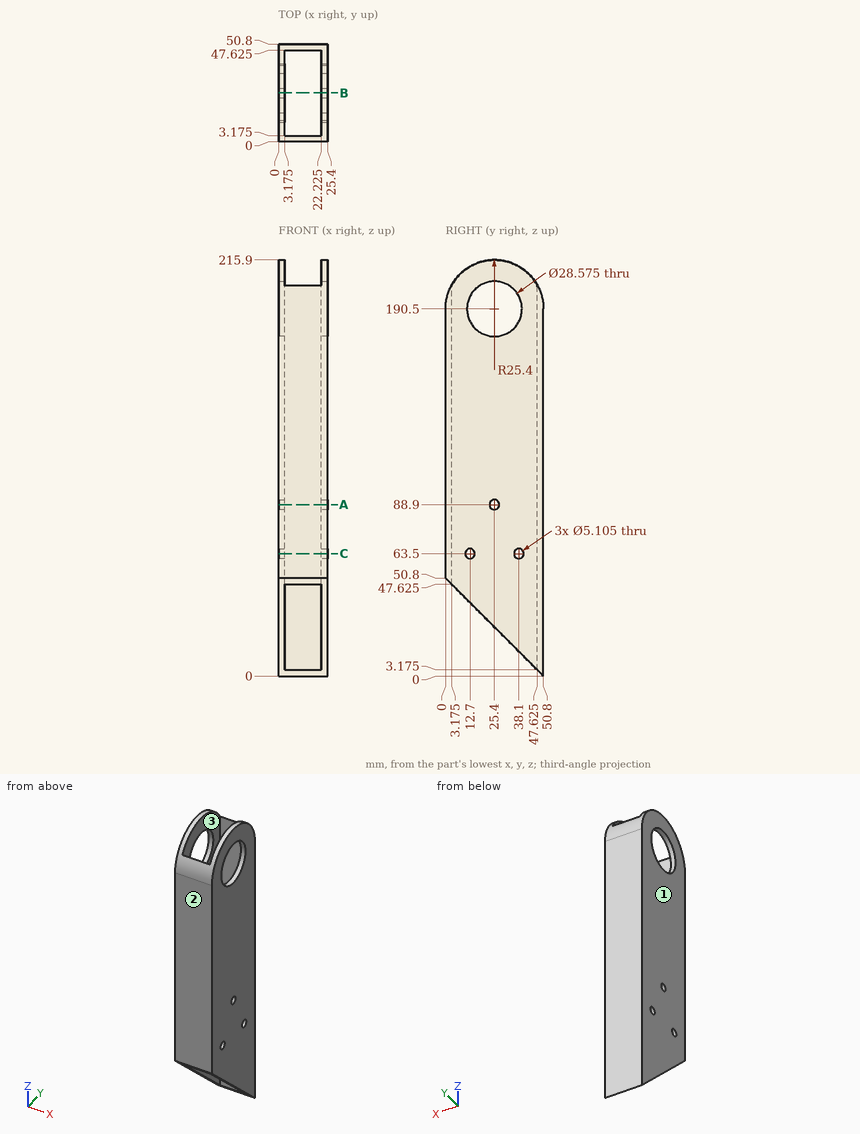
Input: dimensioned drawing with shaded views. Units: mm. Origin: part minimum x, y, z. Coordinates: 2 decimals unless noted, no trailing zeros. Loops run counter-clockwise (first coordinate to the right, second up) from the corner with the lowest first, then second, coordinate; pieces in that order, holes last. Notation, with made-up numbers: (-40, 64.5) -> (5, 64.5) arc R35 ccw to (5, 97.5) -> close; hole circle Ø5 at (66.25, 5.5). An arc over 180 degrees is marked (long way). Use a Markdown table: item, result. Add a question column.
(1) Section query A-A, the plane z = 88.9. Return loops of the section in (x, y) (1 decimal).
(2) Section query C-C, the plane z = 63.5. Return loops of the section in (x, y) (1 decimal).
(3) Section query B-B, the plane y = 25.4. Return loops of the section in (x, z) (1 decimal).
(4) Line query: line 1 along Y through (x, z) = (14.5, 163) (1 decimal); line 2 along X through (y, z) = (24, 168.5) (1 decimal); line 3 along Y through (x, z) = (0.65, 63.5). Output: solid intervals per line, ascending.
(5) Pin query (flat end, axial travel): pin 1 Ø8 at (y, z) = (12.7, 63.5) entering from +X; pin 2 Ø4 at (y, z) = (25.4, 88.9) entering from -X; pin 3 Ø2 at (x, y) = (21.5, 35) entering from -Z. Return the tip coordinate at first contact, or that it passes through.
(6) Mould query, pull axis Y, two halves, no side actions, for the marked faces 1, 2 and 3. Classes: pulls with the +Y half, pulls with the -Y half, needs draft (parallel to the pull), parting line crosses it, or undercut.
Answer:
| question | item | result |
|---|---|---|
| 1 | outline | (0, 0) -> (25.4, 0) -> (25.4, 22.8) -> (22.2, 22.8) -> (22.2, 3.2) -> (3.2, 3.2) -> (3.2, 22.8) -> (0, 22.8) -> close; (0, 28) -> (3.2, 28) -> (3.2, 47.6) -> (22.2, 47.6) -> (22.2, 28) -> (25.4, 28) -> (25.4, 50.8) -> (0, 50.8) -> close |
| 2 | outline | (0, 0) -> (25.4, 0) -> (25.4, 10.1) -> (22.2, 10.1) -> (22.2, 3.2) -> (3.2, 3.2) -> (3.2, 10.1) -> (0, 10.1) -> close; (0, 15.3) -> (3.2, 15.3) -> (3.2, 35.5) -> (0, 35.5) -> close; (0, 40.7) -> (3.2, 40.7) -> (3.2, 47.6) -> (22.2, 47.6) -> (22.2, 40.7) -> (25.4, 40.7) -> (25.4, 50.8) -> (0, 50.8) -> close; (22.2, 15.3) -> (25.4, 15.3) -> (25.4, 35.5) -> (22.2, 35.5) -> close |
| 3 | outline | (0, 25.4) -> (3.2, 25.4) -> (3.2, 86.3) -> (0, 86.3) -> close; (0, 91.5) -> (3.2, 91.5) -> (3.2, 176.2) -> (0, 176.2) -> close; (0, 204.8) -> (3.2, 204.8) -> (3.2, 215.9) -> (0, 215.9) -> close; (22.2, 25.4) -> (25.4, 25.4) -> (25.4, 86.3) -> (22.2, 86.3) -> close; (22.2, 91.5) -> (25.4, 91.5) -> (25.4, 176.2) -> (22.2, 176.2) -> close; (22.2, 204.8) -> (25.4, 204.8) -> (25.4, 215.9) -> (22.2, 215.9) -> close |
| 4 | line 1 | y = 0 to 3.2, 47.6 to 50.8 |
| 4 | line 2 | x = 0 to 3.2, 22.2 to 25.4 |
| 4 | line 3 | y = 0 to 10.15, 15.25 to 35.55, 40.65 to 50.8 |
| 5 | pin 1 | stops at x = 25.4 |
| 5 | pin 2 | passes through |
| 5 | pin 3 | stops at z = 15.11 |
| 6 | face 1 | needs draft |
| 6 | face 2 | pulls with the -Y half |
| 6 | face 3 | undercut |
